Could you check a few things on this model? Use its own coordinates, in mm. Coordinates: 2 decimals unless noted, no trailing zeros. Loops run counter-clockwise (first coordinate to the right, second up) from the corner with the lowest first, then second, coordinate; pieces in that order, holes last. Notation, with made-up numbers: M -24,59.25 L -1,59.25 A32 ccw -1,94.25 Z; hole C 67,52.25 d8. An arc over 180 degrees is marked long. Return JSON: item names as keys, results as strings. Group by question number.
Autodesk Inventor part; units mm, degrees
ref_plane "工作平面1" through (0, 0, 42) normal (0, 0, 1) x (1, 0, 0)
ref_plane "工作平面2" through (1226.4, -727, 42) normal (0.3899335, 0.920843, 0) x (-0.920843, 0.3899335, 0)
ref_plane "YZ Plane" through (0, 0, 0) normal (1, 0, 0) x (0, 1, 0)
ref_plane "工作平面1" through (0, 0, 42) normal (0, 0, 1) x (1, 0, 0)
sketch "草图1" plane through (0, 0, 42) normal (0, 0, 1) x (1, 0, 0)
  line L0 (0, 0) -> (60, 0)
  line L1 (60, 0) -> (60, -1169.8)
  line L2 (60, -1169.8) -> (0, -1169.8)
  line L3 (0, -1169.8) -> (0, 0)
  line L4 (0, -80.6) -> (60, -80.6)
  line L5 (0, -191.9) -> (60, -191.9)
  line L6 (0, -276.5) -> (60, -276.5)
  line L7 (0, -335.9) -> (60, -335.9)
  line L8 (0, -420.6) -> (60, -420.6)
  line L9 (0, -550.6) -> (60, -550.6)
  line L10 (0, -677.8) -> (60, -677.8)
  line L11 (0, -782.9) -> (60, -782.9)
  line L12 (0, -839.5) -> (60, -839.5)
  line L13 (0, -923.6) -> (60, -923.6)
  line L14 (0, -1007.7) -> (60, -1007.7)
  line L15 (0, -1091.2) -> (60, -1091.2)
  line L16 (60, 0) -> (118.4, 0)
  line L17 (118.4, 0) -> (118.4, -23.7)
  line L18 (118.4, -23.7) -> (83.4, -23.7)
  line L19 (83.4, -23.7) -> (83.4, -79.7)
  line L20 (83.4, -79.7) -> (118.4, -79.7)
  line L21 (118.4, -79.7) -> (118.4, -137.6)
  line L22 (118.4, -137.6) -> (83.4, -137.6)
  line L23 (83.4, -137.6) -> (83.4, -276.5)
  line L24 (83.4, -276.5) -> (142.9, -276.5)
  line L25 (142.9, -276.5) -> (142.9, -379.5)
  line L26 (83.4, -276.5) -> (83.4, -379.5)
  line L27 (83.4, -379.5) -> (142.9, -379.5)
  line L28 (142.9, -379.5) -> (142.9, -463)
  line L29 (142.9, -463) -> (83.4, -463)
  line L30 (83.4, -463) -> (83.4, -379.5)
  line L31 (142.9, -463) -> (142.9, -566.2)
  line L32 (142.9, -566.2) -> (83.4, -566.2)
  line L33 (83.4, -566.2) -> (83.4, -463)
  line L34 (142.9, -566.2) -> (146.7, -566.2)
  line L35 (146.7, -566.2) -> (146.7, -616.2)
  line L36 (146.7, -616.2) -> (192.5, -616.2)
  line L37 (192.5, -616.2) -> (192.5, -673.2)
  line L38 (192.5, -616.2) -> (342.5, -616.2)
  line L39 (342.5, -616.2) -> (342.5, -673.2)
  line L40 (342.5, -673.2) -> (143.4, -673.2)
  line L41 (143.4, -673.2) -> (83.4, -673.2)
  line L42 (83.4, -673.2) -> (83.4, -1092.3)
  line L43 (83.4, -1092.3) -> (143.4, -1092.3)
  line L44 (143.4, -1092.3) -> (143.4, -673.2)
  line L45 (83.4, -754.3) -> (143.4, -754.3)
  line L46 (143.4, -837.8) -> (83.4, -837.8)
  line L47 (83.4, -893.6) -> (143.4, -893.6)
  line L48 (143.4, -978.3) -> (83.4, -978.3)
  line L49 (60, -1169.8) -> (188.1, -1169.8)
  line L50 (188.1, -1169.8) -> (188.1, -1092.3)
  line L51 (188.1, -1092.3) -> (143.4, -1092.3)
  line L52 (83.4, -1092.3) -> (83.4, -1117.3)
  line L53 (83.4, -1117.3) -> (188.1, -1117.3)
  line L54 (98.6, -1092.3) -> (98.6, -1117.3)
  line L55 (114.5, -1092.3) -> (114.5, -1117.3)
  line L56 (143.4, -1092.3) -> (143.4, -1117.3)
  line L57 (166.2, -1092.3) -> (166.2, -1117.3)
  line L58 (188.1, -1163.6) -> (336, -1163.6)
  line L59 (188.1, -1137.1) -> (336, -1137.1)
  line L60 (336, -1137.1) -> (336, -1163.6)
  line L61 (342.5, -616.2) -> (398.5, -616.2)
  line L62 (342.5, -673.2) -> (393, -673.2)
  line L63 (393, -673.2) -> (393, -1136.7)
  line L64 (393, -1136.7) -> (393, -1141.7)
  line L65 (393, -1136.7) -> (336, -1137.1)
  line L66 (336, -1163.6) -> (393, -1163.6)
  line L67 (393, -1163.6) -> (393, -1158.6)
  line L68 (393, -1163.6) -> (393, -1188.1)
  line L69 (393, -1188.1) -> (417, -1188.1)
  line L70 (417, -1188.1) -> (542.5, -1188.1)
  line L71 (542.5, -1188.1) -> (542.5, -1127.7)
  line L72 (417, -1188.1) -> (417, -1127.7)
  line L73 (417, -1127.7) -> (542.5, -1127.7)
  line L74 (542.5, -1127.7) -> (542.5, -896.8)
  line L75 (542.5, -896.8) -> (542.5, -786.2)
  line L76 (542.5, -786.2) -> (542.5, -673.6)
  line L77 (542.5, -673.6) -> (393, -673.2)
  line L78 (417, -1127.7) -> (417, -896.8)
  line L79 (417, -896.8) -> (542.5, -896.8)
  line L80 (417, -896.8) -> (417.2959, -786.2)
  line L81 (417.2959, -786.2) -> (542.5, -786.2)
  line L82 (417.2959, -786.2) -> (417.5981, -673.2658)
  line L83 (398.5, -499.2) -> (398.5, -384.2)
  line L84 (398.5, -616.2) -> (398.5, -499.2)
  line L85 (398.5, -616.2) -> (458.5, -616.2)
  line L86 (458.5, -616.2) -> (458.5, -384.2)
  line L87 (458.5, -384.2) -> (398.5, -384.2)
  line L88 (398.5, -499.2) -> (458.5, -499.2)
  line L89 (398.5, -441.7) -> (458.5, -441.7)
  line L90 (458.5, -384.2) -> (458.5, -354.2)
  line L91 (458.5, -354.2) -> (482.5, -369.2)
  line L92 (482.5, -369.2) -> (482.5, -384.2)
  line L93 (482.5, -384.2) -> (542.5, -384.2)
  line L94 (542.5, -384.2) -> (542.5, -413.6)
  line L95 (542.5, -413.6) -> (542.5, -443.7)
  line L96 (542.5, -443.7) -> (542.5, -498.7)
  line L97 (542.5, -498.7) -> (542.5, -616.2)
  line L98 (542.5, -413.6) -> (501.5, -413.6)
  line L99 (542.5, -443.7) -> (482.5, -443.7)
  line L100 (542.5, -616.2) -> (482.5, -616.2)
  line L101 (542.5, -498.7) -> (482.5, -498.7)
  line L102 (482.5, -410.1) -> (501.5, -410.1)
  line L103 (501.5, -410.1) -> (501.5, -423.1)
  line L104 (501.5, -423.1) -> (482.5, -423.1)
  line L105 (482.5, -384.2) -> (482.5, -410.1)
  line L106 (482.5, -423.1) -> (482.5, -616.2)
  line L107 (542.5, -616.2) -> (727.5, -616.2)
  line L108 (727.5, -616.2) -> (727.5, -673.6)
  line L109 (727.5, -673.6) -> (542.5, -673.6)
  line L110 (578, -673.6) -> (578, -726.6)
  line L111 (578, -726.6) -> (605, -726.6)
  line L112 (605, -726.6) -> (605, -673.6)
  line L113 (727.5, -673.6) -> (727.5, -726.6)
  line L114 (727.5, -726.6) -> (700.5, -726.6)
  line L115 (700.5, -726.6) -> (700.5, -673.6)
  line L116 (442.5, -384.2) -> (442.5, -354.2)
  line L117 (442.5, -354.2) -> (458.5, -354.2)
  line L118 (398.5, -384.2) -> (384.5, -384.2)
  line L119 (384.5, -384.2) -> (384.5, -354.2)
  line L120 (384.5, -354.2) -> (400.5, -354.2)
  line L121 (400.5, -354.2) -> (400.5, -384.2)
  line L122 (727.5, -616.2) -> (765.5, -616.2)
  line L123 (765.5, -616.2) -> (825.5, -616.2)
  line L124 (765.5, -616.2) -> (765.5, -504.2)
  line L125 (765.5, -504.2) -> (765.5, -444.2)
  line L126 (765.5, -444.2) -> (825.5, -444.2)
  line L127 (825.5, -444.2) -> (825.5, -504.2)
  line L128 (825.5, -504.2) -> (825.5, -616.2)
  line L129 (825.5, -504.2) -> (765.5, -504.2)
  line L130 (825.5, -444.2) -> (849.2, -444.2)
  line L131 (849.2, -444.2) -> (849.2, -450.2)
  line L132 (849.2, -450.2) -> (868.2, -450.2)
  line L133 (868.2, -450.2) -> (868.2, -502.2)
  line L134 (868.2, -502.2) -> (849.2, -502.2)
  line L135 (849.2, -502.2) -> (849.2, -450.2)
  line L136 (849.2, -502.2) -> (849.2, -506.7)
  line L137 (849.2, -506.7) -> (909.2, -506.7)
  line L138 (909.2, -506.7) -> (909.2, -613.1)
  line L139 (909.2, -613.1) -> (849.2, -613.1)
  line L140 (849.2, -613.1) -> (849.2, -506.7)
  line L141 (727.5, -673.6) -> (765.5, -673.6)
  line L142 (765.5, -673.6) -> (765.5, -786.6)
  line L143 (765.5, -786.6) -> (825.5, -786.6)
  line L144 (825.5, -786.6) -> (825.5, -673.6)
  line L145 (825.5, -673.6) -> (765.5, -673.6)
  line L146 (765.5, -786.6) -> (765.5, -897.6)
  line L147 (765.5, -897.6) -> (825.5, -897.6)
  line L148 (825.5, -897.6) -> (825.5, -786.6)
  line L149 (765.5, -897.6) -> (765.5, -1008.6)
  line L150 (765.5, -1008.6) -> (825.5, -1008.6)
  line L151 (825.5, -1008.6) -> (825.5, -897.6)
  line L152 (765.5, -1008.6) -> (765.5, -1125.1)
  line L153 (765.5, -1125.1) -> (825.5, -1125.1)
  line L154 (825.5, -1125.1) -> (825.5, -1008.6)
  line L155 (765.5, -1125.1) -> (765.5, -1174.6)
  line L156 (765.5, -1174.6) -> (825.5, -1174.6)
  line L157 (825.5, -1174.6) -> (825.5, -1125.1)
  line L158 (825.5, -1174.6) -> (849.2, -1174.6)
  line L159 (849.2, -613.1) -> (849.2, -623.1)
  line L160 (849.2, -623.1) -> (916.2, -623.1)
  line L161 (916.2, -623.1) -> (916.2, -626.6)
  line L162 (849.2, -623.1) -> (849.2, -668.1)
  line L163 (849.2, -668.1) -> (916.2, -668.1)
  line L164 (916.2, -668.1) -> (916.2, -664.6)
  line L165 (849.2, -668.1) -> (849.2, -681.1)
  line L166 (849.2, -681.1) -> (849.2, -1050.1)
  line L167 (849.2, -1050.1) -> (909.2, -1050.1)
  line L168 (909.2, -1050.1) -> (909.2, -1091.6)
  line L169 (909.2, -1091.6) -> (909.2, -1121.1)
  line L170 (909.2, -1121.1) -> (849.2, -1121.1)
  line L171 (849.2, -1121.1) -> (849.2, -1050.1)
  line L172 (909.2, -1091.6) -> (849.2, -1091.6)
  line L173 (849.2, -1174.6) -> (849.2, -1121.1)
  line L174 (849.2, -1174.6) -> (1031.2, -1174.6)
  line L175 (1031.2, -1121.1) -> (909.2, -1121.1)
  line L176 (1031.2, -1121.1) -> (1031.2, -1174.6)
  line L177 (916.2, -626.6) -> (1226.4, -727) construction
  arc A0 (1226.4, -727) -> (916.2, -626.6) centre (761.993, -1632.4479) ccw
  line L178 (916.2, -664.6) -> (1213.4, -757.7) construction
  arc A1 (1213.4, -757.7) -> (916.2, -664.6) centre (605.6007, -2177.0365) ccw
  line L179 (1226.4, -727) -> (1213.4, -757.7)
  line L180 (1226.4, -727) -> (1239.7468, -733.8456)
  line L181 (1213.4, -757.7) -> (1226.7468, -764.5456)
  line L182 (1239.7468, -733.8456) -> (1237.0998, -739.0064)
  line L183 (1226.7468, -764.5456) -> (1229.3938, -759.3849)
  dimension "d1" = 60
  dimension "d2" = 80.6
  dimension "d3" = 111.3
  dimension "d4" = 84.6
  dimension "d5" = 59.4
  dimension "d6" = 84.7
  dimension "d7" = 130
  dimension "d8" = 127.2
  dimension "d9" = 105.1
  dimension "d10" = 56.6
  dimension "d11" = 84.1
  dimension "d12" = 84.1
  dimension "d13" = 83.5
  dimension "d14" = 78.6
  dimension "d15" = 58.4
  dimension "d16" = 23.7
  dimension "d17" = 35
  dimension "d18" = 56
  dimension "d19" = 57.9
  dimension "d20" = 35
  dimension "d21" = 138.9
  dimension "d22" = 59.5
  dimension "d23" = 103
  dimension "d24" = 83.5
  dimension "d25" = 103.2
  dimension "d26" = 59.5
  dimension "d27" = 3.8
  dimension "d28" = 50
  dimension "d29" = 45.8
  dimension "d30" = 57
  dimension "d31" = 150
  dimension "d32" = 57
  dimension "d33" = 199.1
  dimension "d34" = 60
  dimension "d36" = 81.1
  dimension "d37" = 83.5
  dimension "d38" = 55.8
  dimension "d39" = 84.7
  dimension "d40" = 114
  dimension "d41" = 128.1
  dimension "d42" = 25
  dimension "d43" = 15.2
  dimension "d44" = 15.9
  dimension "d45" = 28.9
  dimension "d46" = 22.8
  dimension "d47" = 21.9
  dimension "d48" = 147.9
  dimension "d49" = 6.2
  dimension "d50" = 26.5
  dimension "d51" = 56
  dimension "d52" = 50.5
  dimension "d53" = 463.5
  dimension "d54" = 5
  dimension "d55" = 5
  dimension "d56" = 24.5
  dimension "d57" = 24
  dimension "d58" = 125.5
  dimension "d59" = 60.4
  dimension "d60" = 230.9
  dimension "d61" = 110.6
  dimension "d62" = 112.6
  dimension "d64" = 117
  dimension "d65" = 115
  dimension "d66" = 60
extrude "拉伸1" add sketch "草图1" against normal blind 1 contours L108 L122 L123 L128 L127 L130 L131 L135 L136 L140 L159 L162 L165 L166 L171 L173 L158 L157 L154 L151 L148 L144 L145 L141 | L145 L144 L143 L142 | L124 L129 L128 L123 | L143 L148 L147 L146 | L125 L126 L127 L129 | L147 L151 L150 L149 | L150 L154 L153 L152 | L153 L157 L156 L155 | L132 L133 L134 L135 | L173 L170 L175 L176 L174 | L137 L138 L139 L140 | L171 L172 L169 L170 | L171 L167 L168 L172 | L160 L161 A0 L179 A1 L164 L163 L162
sketch "草图2" plane through (765.5, -1174.6, 42) normal (0, -1, 0) x (1, 0, 0)
  line L0 (265.7, 0) -> (265.7, -1) construction
  line L1 (265.7, -0.5) -> (280.7, 7)
  line L2 (265.7, -0.5) -> (265.7, -0.1)
  line L3 (265.7, -0.1) -> (280.7, 7.4)
  line L4 (280.7, 7.4) -> (280.7, 7)
  point P0 (-765.5, -42)
  dimension "d135" = 7.5
  dimension "d137" = 15
  dimension "d138" = 0.4
extrude "拉伸2" add sketch "草图2" against normal up to surface (53.5 mm away)
ref_plane "工作平面2" through (1226.4, -727, 42) normal (0.3899335, 0.920843, 0) x (-0.920843, 0.3899335, 0)
sketch "草图3" plane through (1226.4, -727, 42) normal (0.3899335, 0.920843, 0) x (-0.920843, 0.3899335, 0)
  line L0 (0, 0) -> (0, -1) construction
  line L1 (0, -0.5) -> (-15, 7)
  line L2 (0, -0.5) -> (0, -0.1)
  line L3 (0, -0.1) -> (-15, 7.4)
  line L4 (-15, 7.4) -> (-15, 7)
  point P0 (1412.8035, -42)
  dimension "d141" = 7.5
  dimension "d144" = 15
  dimension "d145" = 0.4
extrude "拉伸3" add sketch "草图3" against normal blind 33.4
properties part number "LabVIEWM0.5"
(1) If I drill on L1, parallel to Z at x = 794, y = -1022; L2, parallel to Y at x = 1102, z = 41.75, over which ranges is the centre line in solid material (lowest first)? Write a range as [from, to].
(2) We'd pull the mould along X, two halves only. Please class faces 1 (the face through (1077.527, -665.004, 41.507)), 2 (the face through (1069.237, -704.292, 41.507)), 3 (the face through (1038.6, -1148.2, 45.6)): +X half, -X half, draft (parallel to the pull), parting line (faces both ways), or undercut.
(3) Will these pins go through, and if not, where does the flat tip stop? P1, Ø1.1, axis at x = 744.5, z = 41.5, coming from the +Y side; P2, Ø1.5, axis at y = -1034, z = 42.5, coming from the +X side; P3, Ø4, axis at x = 786.5, y = -642.5, coming from the +Z side; P4, Ø5, axis at x = 981.5, z = 45.5, coming from the +Y side.
(4) Imagine slicing it at C-C, the plane y = -819. Write out the boundary of the cut face in (x, z), then the cut area to 3 significant figures.
(5) Imagine slicing it at D-D, the plane x = 774.5. Write out the boundary of the cut face in (y, z).
(6) Imagine slicing it at B-B, the plane x = 988.5. Write out the boundary of the cut face in (y, z), then the cut area to 3 significant figures.
(7) Imagine slicing it at A-A, the plane z = 46. Write out the boundary of the cut face in (x, y).
Checks:
{
 "1": {"L1": "[41, 42]", "L2": "[-715.01, -673.33]"},
 "2": {"face 1": "+X half", "face 2": "undercut", "face 3": "-X half"},
 "3": {"P1": "y = -616.2", "P2": "x = 849.2", "P3": "z = 42", "P4": "through"},
 "4": {"outline": "M 765.5,41 L 849.2,41 L 849.2,42 L 765.5,42 Z", "area": "83.7 mm²"},
 "5": {"outline": "M -1174.6,41 L -444.2,41 L -444.2,42 L -1174.6,42 Z"},
 "6": {"outline": "M -1174.6,41 L -1121.1,41 L -1121.1,42 L -1174.6,42 Z; M -681.27,41 L -640.38,41 L -640.38,42 L -681.27,42 Z", "area": "94.4 mm²"},
 "7": {"outline": "M 1039.4,-1174.6 L 1040.2,-1174.6 L 1040.2,-1121.1 L 1039.4,-1121.1 Z; M 1220.93,-760.95 L 1221.66,-761.27 L 1234.69,-730.51 L 1233.95,-730.2 Z"}
}
